from build123d import *
from build123d.topology import SkipClean

# Parameters (mm, degrees)
ESQUISSE1_R             = 6
BOSS_EXTRU_1_DEPTH      = 5
BOSS_EXTRU_2_REACH      = 21.849
BOSS_EXTRU_2_END_RADIUS = 6
BOSS_EXTRU_2_START      = 10
ESQUISSE4_R             = 0.95
ENL_V_MAT_EXTRU_1_DEPTH = 2
ESQUISSE5_R             = 0.95
ENL_V_MAT_EXTRU_2_DEPTH = 8


with BuildPart() as part:
    # Esquisse1 → Boss.-Extru.1 (new body)
    with BuildSketch(Plane(origin=(0, 0, 0), x_dir=(1, 0, 0), z_dir=(0, 1, 0))):
        with Locations(Location((0, 0, 0), (0, 0, 270))):
            Circle(ESQUISSE1_R)
        with BuildLine():
            Line((-2.076655966, 2.5), (2.076655966, 2.5))
            ThreePointArc((2.076655966, 2.5), (0, -3.25), (-2.076655966, 2.5))
        make_face(mode=Mode.SUBTRACT)
    extrude(amount=BOSS_EXTRU_1_DEPTH)

    # Boss.-Extru.2: up to this cylinder (the profile starts outside it)
    with SkipClean():  # the faces are left unmerged after this step: merging them gives an invalid solid
        boss_extru_2_end = Plane(origin=(0, 2.733375, 0), z_dir=(0, -1, 0)) * Cylinder(BOSS_EXTRU_2_END_RADIUS, 56.698, mode=Mode.PRIVATE)
        # Esquisse3 → Boss.-Extru.2 (add, up to the surface)
        with BuildSketch(Plane(origin=(0, 0, 0), x_dir=(0, 0, -1), z_dir=(1, 0, 0)).offset(BOSS_EXTRU_2_START), mode=Mode.PRIVATE) as boss_extru_2_sk1:
            with BuildLine():
                Line((-2.5, 2.5), (-2.5, 5))
                Line((-2.5, 5), (2.5, 5))
                Line((2.5, 5), (2.5, 2.5))
                ThreePointArc((2.5, 2.5), (0, 0), (-2.5, 2.5))
            make_face()
        boss_extru_2_tool1 = extrude(boss_extru_2_sk1.sketch, amount=-BOSS_EXTRU_2_REACH, mode=Mode.PRIVATE) - boss_extru_2_end
        add(boss_extru_2_tool1.solids().sort_by_distance((10, 2.733375, 0))[0])

    # Esquisse4 → Enl_v. mat.-Extru.1 (cut)
    with SkipClean():  # the faces are left unmerged after this step: merging them gives an invalid solid
        with BuildSketch(Plane(origin=(10, 0, 0), x_dir=(0, 0, -1), z_dir=(1, 0, 0))):
            with Locations((0, 2)):
                Circle(ESQUISSE4_R)
        extrude(amount=-ENL_V_MAT_EXTRU_1_DEPTH, mode=Mode.SUBTRACT)

    # Esquisse5 → Enl_v. mat.-Extru.2 (cut)
    with SkipClean():  # the faces are left unmerged after this step: merging them gives an invalid solid
        with BuildSketch(Plane.XY):
            with Locations((0, 2.5)):
                Circle(ESQUISSE5_R)
        extrude(amount=-ENL_V_MAT_EXTRU_2_DEPTH, mode=Mode.SUBTRACT)


solid = part.part
Input: part model. Units: mm. Frame: model coordinates. A direction names the side the tool comes from. Round coordinates to 2 decimals unless told otherwise and drop trailing zeros. Loops run counter-clockwise (first coordinate to the right, second up) from the corner with the lowest first, then second, coordinate; pieces in that order, holes last. Notation, with made-up numbers: M 2,76 L 8,76 A24 cw 8,90 Z; hole C -10,-13.5 d11. An arc over 180 degrees is marked long. Answer as CSV lines item,"result". Start each with the question number.
(1) Section B-B, the plane x = 9. Output: boundary loops of the cut face in (y, z), plus the area to 3 significant figures.
(2) Section C-C, the plane x = -2.5. Output: boundary loops of the cut face in (y, z), plus the area to 3 significant figures.
(3) Line query: line 1 (Y direction, x = 0, z = -3.5); line 2 (Z direction, x = 0, y = 3.7); line 3 (X direction, y = 3.85, z = 0). Output: solid intervals per line, ascending. Write a range as [from, to].
(4) Draft query along Y for faces 6 (the flat face through (0, 0, -3)), 7 (the flat face through (-1, 2, -2.5)), 8 (the cylindrical face through (9.014, 2.942, 0.124)). Return one class per face: released by +Y, released by -Y, zero draft, split by the parting line, or undercut.
(5) First-contact query: pin 1 (2.5 mm diameter, centred on x = 0, y = 2.5, fed in from -Z); pin 2 (1 mm diameter, centred on x = -2, y = 4, fed in from +Z); pin 3 (1.5 mm diameter, centred on x = -2, y = 2, fed in from -Z); pin 4 (0.6 mm diameter, centred on y = 2.5, z = 0, fed in from +X). Flat tips, straight axial feed; report the tip coordinate or a pass-through.
(6) Reachability of faces 1 (the flat face through (8, 4, 2.5)), 2 (the cylindrical face through (8, 0, 0)), 3 (the cylindrical face through (-0.124, 3.442, -4.226)), 4 (the flat face through (8, 4, -2.5)), 5 (the flat face through (8, 2, 0)) from +Z, -Z, +X, -X, +Y, -Y: full face, straight path, thin tool, end or side. Return the list, or none.
(7) Section D-D, the plane y = 2. Output: boundary loops of the cut face in (x, z).
(8) Section A-A, the plane z = 2. Output: boundary loops of the cut face in (x, y).
Values found:
1,outline,"M 2.5,-2.5 L 5,-2.5 L 5,2.5 L 2.5,2.5 A2.5 ccw Z; hole C 2,0 d1.9"
1,area,"19.5 mm²"
2,outline,"M 0,-5.45 L 5,-5.45 L 5,-2.08 L 0,-2.08 Z; M 0,2.08 L 5,2.08 L 5,5.45 L 0,5.45 Z"
2,area,"33.8 mm²"
3,line 1,"y = [0, 1.55], [3.45, 5]"
3,line 2,"z = [-6, -2.5], [3.25, 6]"
3,line 3,"x = [-6, -3.25], [3.25, 10]"
4,face 6,"released by -Y"
4,face 7,"zero draft"
4,face 8,"undercut"
5,pin 1,"stops at z = -6"
5,pin 2,"stops at z = 5.81"
5,pin 3,"stops at z = -5.87"
5,pin 4,"stops at x = 8"
6,face 1,"+Z, +X, +Y, -Y"
6,face 2,"+X, -Y"
6,face 3,"-Z"
6,face 4,"-Z, +X, +Y, -Y"
6,face 5,"+X"
7,outline,"M -2.08,-2.5 A3.25 cw long 2.08,-2.5 L 0.81,-2.5 L 0.81,-5.95 A6 ccw 5.48,-2.45 L 10,-2.45 L 10,-0.95 L 8,-0.95 L 8,0.95 L 10,0.95 L 10,2.45 L 5.48,2.45 A6 ccw long -0.81,-5.95 L -0.81,-2.5 Z"
8,outline,"M -5.66,0 L -2.56,0 L -2.56,5 L -5.66,5 Z; M 2.56,0 L 5.66,0 L 5.66,1 L 10,1 L 10,5 L 2.56,5 Z"
